Design review of the part built by this model. Coordinates are the model's own, in mm. Face numbers are marked on the shaded views. A direction names the side the tool comes from. Give positions to 0.01 mm unless a question says otherwise; leave off trailing zeros. Write each loop counter-clockwise with the first axis right and the second up, starting at its lowest first coordinate (ties: lowest second). Pieces come first, ordered by that corner, then holes. Notation, with made-up numbers: (56, -17) -> (66, -17) arc R37 ccw to (66, 22) -> close; hole circle Ø7 at (-18.75, 14). An arc over 180 degrees is marked (long way). Put each result on its own line as item: value. Start each with the question number.
from build123d import *

# Parameters (mm, degrees)
F0_R     = 7.9375
F1_DEPTH = 2.54
F2_R     = 6.35
F3_DEPTH = 12.7
F5_DEPTH = 12.7


with BuildPart() as f1:
    # F0 (on Top) → F1 (new body)
    with BuildSketch(Plane.XY):
        Circle(F0_R)
    extrude(amount=F1_DEPTH)

    # F2 (on face) → F3 (join)
    with BuildSketch(Plane.XY.offset(2.54)):
        Circle(F2_R)
    extrude(amount=F3_DEPTH)

    # F4 (on face) → F5 (cut, through all)
    with BuildSketch(Plane.XY.offset(15.24)):
        with BuildLine():
            Line((1, 4.898979), (-1, 4.898979))
            ThreePointArc((-1, 4.898979), (-3.535534, 3.535534), (-4.898979, 1))
            Line((-4.898979, 1), (-4.898979, -1))
            ThreePointArc((-4.898979, -1), (-3.535534, -3.535534), (-1, -4.898979))
            Line((-1, -4.898979), (1, -4.898979))
            ThreePointArc((1, -4.898979), (3.535534, -3.535534), (4.898979, -1))
            Line((4.898979, -1), (4.898979, 1))
            ThreePointArc((4.898979, 1), (3.535534, 3.535534), (1, 4.898979))
        make_face()
    extrude(amount=-F5_DEPTH, mode=Mode.SUBTRACT)


solid = f1.part
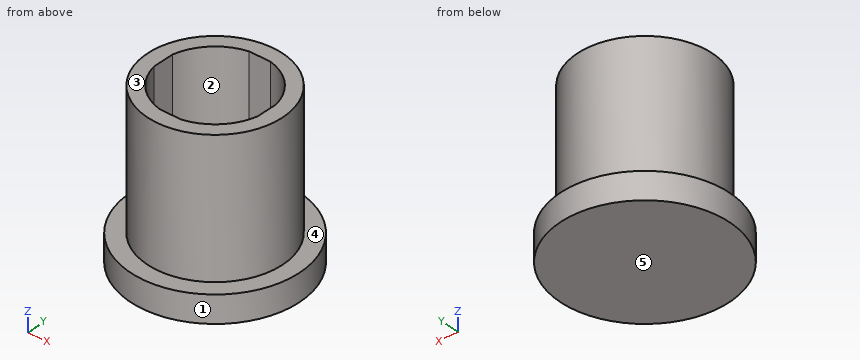
Q1. Machinability: for the marked faces 4 and 5, which of the approach directions +Z, -Z, +X, -X, +Y, -Y give a long, thin tool a straight path to every point of the face, cutting with its end or side? Answer none if there is none.
Q2. To check wall thickness, follow probe 1 along X at (y, z) = (-0.25, 9.75); probe 2 along Z at (x, y) = (-2.5, 6). State the ranges of each line that lie inside material, in increasing order. Write a range as from..to.
Q3. Take a section at B-B on y = 0. Give the boundary of the cut face in (x, z), then the cut area to 3 significant figures.
Q4. For pin 1 (1.6 mm diameter, centred on x = 0.5, z = 12, fed in from +Y); pin 2 (2 mm diameter, centred on y = -0.5, z = 10, fed in from +X); pin 3 (6 mm diameter, centred on x = 5.5, z = 3.5, fed in from +Y), all flat-tipped, find the tip position at first contact; note any pin that passes through.
Q5. Mouldability with a two-part tool opening along Y and no side actions: class the marked faces 1, 2 and 3 as +Y half, -Y half, draft (parallel to the pull), parting line (faces both ways), or undercut.
Q6. Take a section at A-A on z = 3.75. Give the boundary of the cut face in (x, y).
Q7. Take a section at D-D on x = 5.75. Give the boundary of the cut face in (y, z), then the cut area to 3 significant figures.
Result:
1. face 4: +Z
1. face 5: -Z, +X, -X, +Y, -Y
2. probe 1: x = -6.35..-4.9, 4.9..6.35
2. probe 2: z = 0..2.54
3. outline: (-7.94, 0) -> (7.94, 0) -> (7.94, 2.54) -> (6.35, 2.54) -> (6.35, 15.24) -> (4.9, 15.24) -> (4.9, 2.54) -> (-4.9, 2.54) -> (-4.9, 15.24) -> (-6.35, 15.24) -> (-6.35, 2.54) -> (-7.94, 2.54) -> close
3. area: 77.2 mm^2
4. pin 1: stops at y = 6.35
4. pin 2: stops at x = 6.35
4. pin 3: stops at y = 7.48
5. face 1: parting line
5. face 2: undercut
5. face 3: draft
6. outline: circle Ø12.7 at (0, 0); hole (-4.9, -1) arc R5 ccw to (-1, -4.9) -> (1, -4.9) arc R5 ccw to (4.9, -1) -> (4.9, 1) arc R5 ccw to (1, 4.9) -> (-1, 4.9) arc R5 ccw to (-4.9, 1) -> close
7. outline: (-5.47, 0) -> (5.47, 0) -> (5.47, 2.54) -> (2.69, 2.54) -> (2.69, 15.24) -> (-2.69, 15.24) -> (-2.69, 2.54) -> (-5.47, 2.54) -> close
7. area: 96.2 mm^2
